Input: part model. Units: mm. Frame: model coordinates. A direction names the side the tool comes from. Give positions to 0.01 mm unless a question says otherwise; leave off trailing zeros. Answer as a JSON object with one key per item and string values. Group by question number.
(1) Mould query, pull axis Y, two halves, no side actions, for faces 1 (the flat face through (7, 0, -3)), 2 (the cylindrical face through (9.6, 4.5, -3.3)), 3 (the flat face through (0.15, 3, -4)), 4 (the flat face through (7, 6.4, -3)). Classes: +Y half, -Y half, draft (parallel to the pull), parting line (faces both ways), or undercut.
(2) Access query for faces 5 (the cylindrical face through (6.04, 1.66, -4.04)), 6 (the flat face through (11, 5.9, 0.5)), 7 (the flat face through (17.85, 3.2, 0.5)). Directions: +Z, -Z, +X, -X, +Y, -Y. A direction counts if a zero-diameter tool reaches every point of the face in a straight line with its end or side. Return the directions, or none.
(3) Section query A-A (x = 8). Count the separate pieces of the cut face and the enclosed holes in it, plus the area to 3 significant figures.
(4) Pin query (flat end, axial travel): P1, Ø1.1, axis at x = 11.5, z = 0.5, coming from the -Y side; P2, Ø1.2, axis at x = 12.85, y = 4.45, coming from the +Z side; P3, Ø2.5, axis at x = 7.85, y = 1.95, coming from the +Z side. Return the tip coordinate at first contact, or that it passes through.
(5) Material intervals for L1, parallel to X at y = 2, z = 0.25; L2, parallel to X at y = 1.95, z = -3.75; L3, parallel to Y at x = 10.75, z = -3.25, sorted ascending.
```python
from build123d import *

# Parameters (mm, degrees)
BOSS_EXTRUDE1_DEPTH = 6.4
CUT_EXTRUDE1_REACH  = 17
SKETCH2_R           = 0.75
CUT_EXTRUDE2_REACH  = 8.4
SKETCH9_W           = 0.5
SKETCH9_H           = 6.4
SKETCH9_W_2         = 1
SKETCH9_W_3         = 11
SKETCH9_H_2         = 0.5
BOSS_EXTRUDE2_DEPTH = 1
SKETCH10_W          = 10.242926678
SKETCH10_H          = 6.4
CUT_EXTRUDE7_DEPTH  = 0.15


with BuildPart() as part:
    # Sketch1 → Boss-Extrude1 (new body)
    with BuildSketch(Plane(origin=(0, 0, 0), x_dir=(1, 0, 0), z_dir=(0, 1, 0))):
        Polygon((0, 15), (0, 0), (18.850032676, 0), (18.850032676, 10), align=None)
    extrude(amount=BOSS_EXTRUDE1_DEPTH)

    # Cut-Extrude1: up to this plane
    cut_extrude1_end = Plane(origin=(18.850032676, 6.4, -10), z_dir=(-0.256385401, 0, 0.966574636))
    # Sketch2 → Cut-Extrude1 (cut, up to the surface)
    with BuildSketch(Plane.XY, mode=Mode.PRIVATE) as cut_extrude1_sk1:
        with Locations((12.850032676, 4.45)):
            Circle(SKETCH2_R)
    cut_extrude1_tool1 = split(extrude(cut_extrude1_sk1.sketch, amount=-CUT_EXTRUDE1_REACH, mode=Mode.PRIVATE), bisect_by=cut_extrude1_end, keep=Keep.BOTH, mode=Mode.PRIVATE)
    add(cut_extrude1_tool1.solids().sort_by_distance((12.850033, 4.45, 0))[0], mode=Mode.SUBTRACT)
    # Sketch2 → Cut-Extrude1 (cut, up to the surface)
    with BuildSketch(Plane.XY, mode=Mode.PRIVATE) as cut_extrude1_sk2:
        with Locations((12.850032676, 1.95)):
            Circle(SKETCH2_R)
    cut_extrude1_tool2 = split(extrude(cut_extrude1_sk2.sketch, amount=-CUT_EXTRUDE1_REACH, mode=Mode.PRIVATE), bisect_by=cut_extrude1_end, keep=Keep.BOTH, mode=Mode.PRIVATE)
    add(cut_extrude1_tool2.solids().sort_by_distance((12.850033, 1.95, 0))[0], mode=Mode.SUBTRACT)
    # Sketch2 → Cut-Extrude1 (cut, up to the surface)
    with BuildSketch(Plane.XY, mode=Mode.PRIVATE) as cut_extrude1_sk3:
        with Locations((5.350032676, 1.95)):
            Circle(SKETCH2_R)
    cut_extrude1_tool3 = split(extrude(cut_extrude1_sk3.sketch, amount=-CUT_EXTRUDE1_REACH, mode=Mode.PRIVATE), bisect_by=cut_extrude1_end, keep=Keep.BOTH, mode=Mode.PRIVATE)
    add(cut_extrude1_tool3.solids().sort_by_distance((5.350033, 1.95, 0))[0], mode=Mode.SUBTRACT)
    # Sketch2 → Cut-Extrude1 (cut, up to the surface)
    with BuildSketch(Plane.XY, mode=Mode.PRIVATE) as cut_extrude1_sk4:
        with Locations((5.350032676, 4.45)):
            Circle(SKETCH2_R)
    cut_extrude1_tool4 = split(extrude(cut_extrude1_sk4.sketch, amount=-CUT_EXTRUDE1_REACH, mode=Mode.PRIVATE), bisect_by=cut_extrude1_end, keep=Keep.BOTH, mode=Mode.PRIVATE)
    add(cut_extrude1_tool4.solids().sort_by_distance((5.350033, 4.45, 0))[0], mode=Mode.SUBTRACT)
    # Sketch2 → Cut-Extrude1 (cut, up to the surface)
    with BuildSketch(Plane.XY, mode=Mode.PRIVATE) as cut_extrude1_sk5:
        with Locations((7.850032676, 4.45)):
            Circle(SKETCH2_R)
    cut_extrude1_tool5 = split(extrude(cut_extrude1_sk5.sketch, amount=-CUT_EXTRUDE1_REACH, mode=Mode.PRIVATE), bisect_by=cut_extrude1_end, keep=Keep.BOTH, mode=Mode.PRIVATE)
    add(cut_extrude1_tool5.solids().sort_by_distance((7.850033, 4.45, 0))[0], mode=Mode.SUBTRACT)
    # Sketch2 → Cut-Extrude1 (cut, up to the surface)
    with BuildSketch(Plane.XY, mode=Mode.PRIVATE) as cut_extrude1_sk6:
        with Locations((10.350032676, 4.45)):
            Circle(SKETCH2_R)
    cut_extrude1_tool6 = split(extrude(cut_extrude1_sk6.sketch, amount=-CUT_EXTRUDE1_REACH, mode=Mode.PRIVATE), bisect_by=cut_extrude1_end, keep=Keep.BOTH, mode=Mode.PRIVATE)
    add(cut_extrude1_tool6.solids().sort_by_distance((10.350033, 4.45, 0))[0], mode=Mode.SUBTRACT)
    # Sketch2 → Cut-Extrude1 (cut, up to the surface)
    with BuildSketch(Plane.XY, mode=Mode.PRIVATE) as cut_extrude1_sk7:
        with Locations((7.850032676, 1.95)):
            Circle(SKETCH2_R)
    cut_extrude1_tool7 = split(extrude(cut_extrude1_sk7.sketch, amount=-CUT_EXTRUDE1_REACH, mode=Mode.PRIVATE), bisect_by=cut_extrude1_end, keep=Keep.BOTH, mode=Mode.PRIVATE)
    add(cut_extrude1_tool7.solids().sort_by_distance((7.850033, 1.95, 0))[0], mode=Mode.SUBTRACT)
    # Sketch2 → Cut-Extrude1 (cut, up to the surface)
    with BuildSketch(Plane.XY, mode=Mode.PRIVATE) as cut_extrude1_sk8:
        with Locations((10.350032676, 1.95)):
            Circle(SKETCH2_R)
    cut_extrude1_tool8 = split(extrude(cut_extrude1_sk8.sketch, amount=-CUT_EXTRUDE1_REACH, mode=Mode.PRIVATE), bisect_by=cut_extrude1_end, keep=Keep.BOTH, mode=Mode.PRIVATE)
    add(cut_extrude1_tool8.solids().sort_by_distance((10.350033, 1.95, 0))[0], mode=Mode.SUBTRACT)

    # Sketch3 → Cut-Extrude2 (cut, up to next)
    with BuildSketch(Plane(origin=(0, 6.4, 0), x_dir=(1, 0, 0), z_dir=(0, 1, 0)), mode=Mode.PRIVATE) as cut_extrude2_sk1:
        with BuildLine():
            Line((0, 15), (0, 9.242926678))
            add(Edge.make_bspline(
                [(18.850032676, 2.408422132), (9.827679117, 7.423862257), (0, 9.242926678)],
                knots=[2.52003539, 2.52003539, 2.52003539, 2.823158509, 2.823158509, 2.823158509], degree=2, weights=[1, 0.988536516, 1]))
            Line((18.850032676, 2.408422132), (18.850032676, 10))
            Line((18.850032676, 10), (0, 15))
        make_face()
    cut_extrude2_tool1 = extrude(cut_extrude2_sk1.sketch, amount=-CUT_EXTRUDE2_REACH, mode=Mode.PRIVATE) & part.part
    add(cut_extrude2_tool1.solids().sort_by_distance((9.890162, 6.4, -9.301074))[0], mode=Mode.SUBTRACT)

    # Sketch9 → Boss-Extrude2 (add)
    with BuildSketch(Plane.XY):
        with Locations((0.25, 3.2)):
            Rectangle(SKETCH9_W, SKETCH9_H)
        with Locations((18.350032676, 3.2)):
            Rectangle(SKETCH9_W_2, SKETCH9_H)
        with Locations((11.050032676, 6.15)):
            Rectangle(SKETCH9_W_3, SKETCH9_H_2)
        with Locations((11.050032676, 0.25)):
            Rectangle(SKETCH9_W_3, SKETCH9_H_2)
    extrude(amount=BOSS_EXTRUDE2_DEPTH)

    # Sketch10 → Cut-Extrude7 (cut)
    with BuildSketch(Plane.ZY):
        with Locations((-4.121463339, 3.2)):
            Rectangle(SKETCH10_W, SKETCH10_H)
    extrude(amount=-CUT_EXTRUDE7_DEPTH, mode=Mode.SUBTRACT)


solid = part.part
```
Recorded:
{
 "1": {"face 1": "-Y half", "face 2": "undercut", "face 3": "draft", "face 4": "+Y half"},
 "2": {"face 5": "+Z, -Z", "face 6": "+Z", "face 7": "+Z, +Y, -Y"},
 "3": {"separate pieces": "3", "enclosed holes": "0", "area": "25.9 mm^2"},
 "4": {"P1": "stops at y = 0", "P2": "passes through", "P3": "stops at z = 0"},
 "5": {"L1": "x = 0.15 to 0.5, 17.85 to 18.85", "L2": "x = 0.15 to 4.6, 6.1 to 7.1, 8.6 to 9.6, 11.1 to 12.1, 13.6 to 16.31", "L3": "y = 0 to 1.32, 2.58 to 3.82, 5.08 to 6.4"}
}
